from build123d import *

# Parameters (mm, degrees)
SKETCH1_W           = 160
SKETCH1_H           = 5
BOSS_EXTRUDE1_DEPTH = 5
SKETCH2_W           = 15
SKETCH2_H           = 5
CUT_EXTRUDE1_DEPTH  = 2.5
SKETCH3_R           = 1.5
CUT_EXTRUDE2_DEPTH  = 2.5


with BuildPart() as part:
    # Sketch1 → Boss-Extrude1 (new body)
    with BuildSketch(Plane.XY):
        Rectangle(SKETCH1_W, SKETCH1_H)
    extrude(amount=BOSS_EXTRUDE1_DEPTH)

    # Sketch2 → Cut-Extrude1 (cut)
    with BuildSketch(Plane(origin=(0, 2.5, 0), x_dir=(1, 0, 0), z_dir=(0, 1, 0))):
        with Locations((-72.5, -2.5)):
            Rectangle(SKETCH2_W, SKETCH2_H)
        with Locations((72.5, -2.5)):
            Rectangle(SKETCH2_W, SKETCH2_H)
    extrude(amount=-CUT_EXTRUDE1_DEPTH, mode=Mode.SUBTRACT)

    # Sketch3 → Cut-Extrude2 (cut)
    with BuildSketch(Plane(origin=(0, 0, 0), x_dir=(1, 0, 0), z_dir=(0, 1, 0))):
        with Locations(Location((-75.030916446, -2.499854379, 0), (0, 0, 270))):
            Circle(SKETCH3_R)
        with Locations(Location((75.030916446, -2.499854379, 0), (0, 0, 90))):
            Circle(SKETCH3_R)
    extrude(amount=-CUT_EXTRUDE2_DEPTH, mode=Mode.SUBTRACT)


solid = part.part
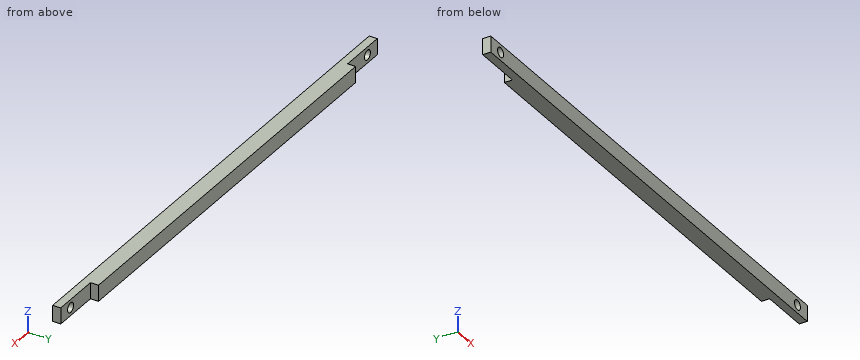
Build history of the part. All positions in model axes, mm. Coordinates: 2 decimals unless noted, no trailing zeros. Order: outer loops, then holes, each group sorted by start corner. A loop starts at its lowest first (then second) coordinate and runs counter-clockwise, first axis right, second up. Notation, with made-up numbers: M 26.25,86 L 63.25,86 A23 cw 63.25,105 Z; hole C 60,-6.75 d10. An arc over 180 degrees is marked long. One line per question, with ' | ' between items. Start each with the question number.
Q1. Probe L1, parallel to X at y = -1.05, z = 2.45; L2, parallel to X at y = -0.3, z = 1.5; L3, parallel to X at y = 1.5, z = 1.75. List the from-to ranges inside material, lowest first. Write a range as from..to.
Q2. Flat gauge pins, fed straight in: pin 1 Ø1.5 at (x, z) = (71, 3) entering from +Y; pin 2 Ø1.2 at (y, z) = (1, 2.5) entering from +X. Where does each tip first touch, or does it go through?
Q3. Saw through at A-A (z = 2.5). List the corners of the cut face in (x, y), then the cut area to 3 significant figures.
Q4. Saw through at B-B (y = -1.45). List the corners of the cut face in (x, z), then the cut area to 3 significant figures.
Check values:
1) L1: x = -80..-76.53, -73.53..73.53, 76.53..80 | L2: x = -80..-76.15, -73.91..73.91, 76.15..80 | L3: x = -65..65
2) pin 1: stops at y = 0 | pin 2: stops at x = 65
3) outline: M -80,-2.5 L -76.53,-2.5 L -76.53,0 L -80,0 Z; M -73.53,-2.5 L 73.53,-2.5 L 73.53,0 L 65,0 L 65,2.5 L -65,2.5 L -65,0 L -73.53,0 Z; M 76.53,-2.5 L 80,-2.5 L 80,0 L 76.53,0 Z | area: 710 mm2
4) outline: M -80,0 L 80,0 L 80,5 L -80,5 Z; hole C -75.03,2.5 d3; hole C 75.03,2.5 d3 | area: 786 mm2
